from build123d import *

# Parameters (mm, degrees)
SKETCH_1_R           = 21
SKETCH_1_R_2         = 20
SKETCH_1_R_3         = 2
EXTRUDE_1_DEPTH      = 8
EXTRUDE_START        = -7
SKETCH_1_3_R         = 20
SKETCH_1_3_R_2       = 2
EXTRUDE_2_DEPTH      = 7
SKETCH_3_R           = 5
CUT_EXTRUDE_10_DEPTH = 25
CUT_EXTRUDE_11_DEPTH = 25
FILLET_8_R           = 2
EXTRUDE_START_2      = -8
EXTRUDE_4_DEPTH      = 8
SKETCH_14_R          = 2
CUT_EXTRUDE_13_DEPTH = 8
SKETCH_15_W          = 10
SKETCH_15_H          = 10
CUT_EXTRUDE_14_DEPTH = 20
CUT_EXTRUDE_START    = 26
SKETCH_16_R          = 20
CUT_EXTRUDE_15_DEPTH = 26
CUT_EXTRUDE_16_DEPTH = 4.5
CUT_EXTRUDE_17_DEPTH = 10
FILLET_9_R           = 1
FILLET_10_R          = 3


with BuildPart() as part:
    # Sketch 1 → Extrude 1 (new body)
    # profile 1 of 2: a face of its own
    with BuildSketch(Plane.XY):
        Circle(SKETCH_1_R)
        Circle(SKETCH_1_R_2, mode=Mode.SUBTRACT)
    # profile 2 of 2: a face of its own
    with BuildSketch(Plane.XY):
        Circle(SKETCH_1_R_2)
        with Locations((8, -13.856406461)):
            Circle(SKETCH_1_R_3, mode=Mode.SUBTRACT)
        with Locations((8, 13.856406461)):
            Circle(SKETCH_1_R_3, mode=Mode.SUBTRACT)
        with Locations((-16, 0)):
            Circle(SKETCH_1_R_3, mode=Mode.SUBTRACT)
    extrude(amount=EXTRUDE_1_DEPTH)

    # Sketch 1_3 → Extrude 2 (add)
    with BuildSketch(Plane.XY.offset(EXTRUDE_START)):
        Circle(SKETCH_1_3_R)
        with Locations((8, -13.856406461)):
            Circle(SKETCH_1_3_R_2, mode=Mode.SUBTRACT)
        with Locations((8, 13.856406461)):
            Circle(SKETCH_1_3_R_2, mode=Mode.SUBTRACT)
        with Locations((-16, 0)):
            Circle(SKETCH_1_3_R_2, mode=Mode.SUBTRACT)
    extrude(amount=EXTRUDE_2_DEPTH)

    # Sketch 3 → Cut-Extrude 10 (cut)
    with BuildSketch(Plane(origin=(0, 0, -7), x_dir=(-1, 0, 0), z_dir=(0, 0, -1))):
        Circle(SKETCH_3_R)
    extrude(amount=-CUT_EXTRUDE_10_DEPTH, mode=Mode.SUBTRACT)

    # Sketch 7 → Cut-Extrude 11 (cut)
    with BuildSketch(Plane(origin=(0, 0, -7), x_dir=(-1, 0, 0), z_dir=(0, 0, -1))):
        with BuildLine():
            Line((0, 13.5), (0, 18))
            ThreePointArc((0, 18), (9, 15.588457268), (15.588457268, 9))
            Line((15.588457268, 9), (11.691342951, 6.75))
            ThreePointArc((11.691342951, 6.75), (6.75, 11.691342951), (0, 13.5))
        make_face()
        with BuildLine():
            Line((11.691342951, -6.75), (15.588457268, -9))
            ThreePointArc((15.588457268, -9), (9, -15.588457268), (0, -18))
            Line((0, -18), (0, -13.5))
            ThreePointArc((0, -13.5), (6.75, -11.691342951), (11.691342951, -6.75))
        make_face()
        with BuildLine():
            Line((-11.691342951, -6.75), (-15.588457268, -9))
            ThreePointArc((-15.588457268, -9), (-18, 0), (-15.588457268, 9))
            Line((-15.588457268, 9), (-11.691342951, 6.75))
            ThreePointArc((-11.691342951, 6.75), (-13.5, 0), (-11.691342951, -6.75))
        make_face()
    extrude(amount=-CUT_EXTRUDE_11_DEPTH, mode=Mode.SUBTRACT)

    # Fillet 8
    fillet_8_edges = [part.edges().sort_by_distance(p)[0] for p in [
        (15.588457268, -9, 0.5),
        (15.588457268, 9, 0.5),
        (11.691342951, 6.75, 0.5),
        (11.691342951, -6.75, 0.5),
        (-15.588457268, -9, 0.5),
        (0, -18, 0.5),
        (0, -13.5, 0.5),
        (-11.691342951, -6.75, 0.5),
        (0, 18, 0.5),
        (-15.588457268, 9, 0.5),
        (-11.691342951, 6.75, 0.5),
        (0, 13.5, 0.5),
    ]]
    fillet(fillet_8_edges, radius=FILLET_8_R)

    # Sketch 12 → Extrude 4 (add)
    with BuildSketch(Plane.XY.offset(8).offset(EXTRUDE_START_2)):
        with BuildLine():
            Line((95.947368421, 14.970053209), (1.326315789, 20.958074492))
            ThreePointArc((1.326315789, 20.958074492), (20.999544828, 0.138264258), (1.602171257, -20.93879288))
            Line((1.602171257, -20.93879288), (95.75, -14.981238267))
            ThreePointArc((95.75, -14.981238267), (109.999674335, -0.09884255), (95.947368421, 14.970053209))
        make_face()
    extrude(amount=EXTRUDE_4_DEPTH)

    # Sketch 14 → Cut-Extrude 13 (cut)
    with BuildSketch(Plane.XY.offset(8)):
        with Locations((95, 10)):
            Circle(SKETCH_14_R)
        with Locations((105, 0)):
            Circle(SKETCH_14_R)
        with Locations((95, -10)):
            Circle(SKETCH_14_R)
        with Locations((85, 0)):
            Circle(SKETCH_14_R)
    extrude(amount=-CUT_EXTRUDE_13_DEPTH, mode=Mode.SUBTRACT)

    # Sketch 15 → Cut-Extrude 14 (cut)
    with BuildSketch(Plane.XY.offset(8)):
        with Locations((95, 0)):
            Rectangle(SKETCH_15_W, SKETCH_15_H)
    extrude(amount=-CUT_EXTRUDE_14_DEPTH, mode=Mode.SUBTRACT)

    # Sketch 16 → Cut-Extrude 15 (cut)
    with BuildSketch(Plane(origin=(0, 0, 0), x_dir=(-1, 0, 0), z_dir=(0, 0, -1)).offset(CUT_EXTRUDE_START)):
        Circle(SKETCH_16_R)
    extrude(amount=-CUT_EXTRUDE_15_DEPTH, mode=Mode.SUBTRACT)

    # Sketch 17 → Cut-Extrude 16 (cut)
    with BuildSketch(Plane.XY.offset(8)):
        Polygon((4.5, -11.835680518), (4.5, -15.877132403), (8, -17.897858345), (11.5, -15.877132403), (11.5, -11.835680518), (8, -9.814954576), align=None)
        Polygon((8, 9.814954576), (11.5, 11.835680518), (11.5, 15.877132403), (8, 17.897858345), (4.5, 15.877132403), (4.5, 11.835680518), align=None)
        Polygon((-12.5, 2.020725942), (-16, 4.041451884), (-19.5, 2.020725942), (-19.5, -2.020725942), (-16, -4.041451884), (-12.5, -2.020725942), align=None)
    extrude(amount=-CUT_EXTRUDE_16_DEPTH, mode=Mode.SUBTRACT)

    # Sketch 13 → Cut-Extrude 17 (cut)
    with BuildSketch(Plane.XY.offset(8)):
        with BuildLine():
            Line((38.858770913, -13.571242245), (68.739124089, -11.680451578))
            ThreePointArc((68.739124089, -11.680451578), (79.70381363, 0), (68.739124089, 11.680451578))
            Line((68.739124089, 11.680451578), (38.858770913, 13.571242245))
            ThreePointArc((38.858770913, 13.571242245), (24.401613936, 0), (38.858770913, -13.571242245))
        make_face()
    extrude(amount=-CUT_EXTRUDE_17_DEPTH, mode=Mode.SUBTRACT)

    # Fillet 9
    fillet_9_edges = [part.edges().sort_by_distance(p)[0] for p in [
        (8, 9.814954576, 5.75),
        (4.5, 11.835680518, 5.75),
        (4.5, 15.877132403, 5.75),
        (8, 17.897858345, 5.75),
        (11.5, 15.877132403, 5.75),
        (11.5, 11.835680518, 5.75),
        (4.5, -11.835680518, 5.75),
        (8, -9.814954576, 5.75),
        (11.5, -11.835680518, 5.75),
        (11.5, -15.877132403, 5.75),
        (8, -17.897858345, 5.75),
        (4.5, -15.877132403, 5.75),
        (-12.5, 2.020725942, 5.75),
        (-12.5, -2.020725942, 5.75),
        (-16, -4.041451884, 5.75),
        (-19.5, -2.020725942, 5.75),
        (-19.5, 2.020725942, 5.75),
        (-16, 4.041451884, 5.75),
    ]]
    fillet(fillet_9_edges, radius=FILLET_9_R)

    # Fillet 10
    fillet_10_edges = [part.edges().sort_by_distance(p)[0] for p in [
        (100, 5, 4),
        (100, -5, 4),
        (90, -5, 4),
        (90, 5, 4),
    ]]
    fillet(fillet_10_edges, radius=FILLET_10_R)


solid = part.part
Work out the finished part from the listing and answer in its coordinate system (mm). A direction names the side the tool comes from. Coordinates: 2 decimals unless noted, no trailing zeros. Loops run counter-clockwise (first coordinate to the right, second up) from the corner with the lowest first, then second, coordinate; pieces in that order, holes last. Notation, with made-up numbers: (-19.5, 35) -> (-7.5, 35) arc R22 cw to (-7.5, 73) -> close; hole circle Ø8 at (-26.5, 15.5). An arc over 180 degrees is marked (long way). Write each question's results on one line, items separated by ' | '. Start each with the question number.
1) Find section C-C on x = 105. Determine the outline of the cut face in (y, z), then the cut area to 3 significant figures.
2) Consider line 1 along Y through (x, z) = (-16, 2.1); line 2 along X through (y, z) = (9.5, 3); line 3 along Y through (x, z) = (95, 5.25). Determine where each line is inside the solid, lowest interval first.
3) Find section A-A on x = 47.5. Determine the outline of the cut face in (y, z), then the cut area to 3 significant figures.
4) Flat-ended cylindrical pins translate along their axes: P1, Ø1, axis at x = 85, y = 14, coming from the -Z side; P2, Ø0.6, axis at y = 15.5, z = 5, coming from the -X side; P3, Ø3, axis at y = -14, z = 5.5, coming from the -X side; P4, Ø1.2, axis at x = 94, z = 3, coming from the +Y side. Find the tip coordinate at first contact, or state that the pin passes through.
5) Find section B-B on z = 5.25. Count the separate pieces of the cut face and the enclosed holes in it, then the cut area to 3 significant figures.
6) For faces 1 (the cylindrical face through (-14.713, 9.297, 4.056)), 2 (the flat face through (10, 12, 3.5)), determine the directions among +Z, -Z, +X, -X, +Y, -Y from which every point of the face is accessible in a straight line to the end or side of a thin tool.
Response values:
1) outline: (-11.18, 0) -> (-2, 0) -> (-2, 8) -> (-11.18, 8) -> close; (2, 0) -> (11.18, 0) -> (11.18, 8) -> (2, 8) -> close | area: 147 mm^2
2) line 1: y = -13.6 to -2, 2 to 13.6 | line 2: x = -18.73 to -14.74, -9.59 to 28.27, 74.84 to 93.06, 96.94 to 106.61 | line 3: y = -15.03 to -12, -8 to -5, 5 to 8, 12 to 15.03
3) outline: (-18.03, 0) -> (-13.02, 0) -> (-13.02, 8) -> (-18.03, 8) -> close; (13.02, 0) -> (18.04, 0) -> (18.04, 8) -> (13.02, 8) -> close | area: 80.2 mm^2
4) P1: stops at z = 0 | P2: stops at x = -14.49 | P3: stops at x = -16.87 | P4: stops at y = 15.13
5) separate pieces: 1 | enclosed holes: 13 | area: 2,650 mm^2
6) face 1: +Z, -Z | face 2: +Z
